Here's how the part is built. I have some questions about the finished solid (model axes, mm). Face numbers are marked on the shaded views. A direction names the side the tool comes from. Round coordinates to 2 decimals unless told otherwise and drop trailing zeros. Order: outer loops, then holes, each group sorted by start corner. A loop starts at its lowest first (then second) coordinate and runs counter-clockwise, first axis right, second up. Notation, with made-up numbers: M 22,-32.75 L 72,-32.75 A25 cw 72,-9.75 Z; hole C -7.5,46.5 d4. An arc over 180 degrees is marked long. Write item = value, one per line. Start each with the question number.
Item 1: I want a section at C-C, the plane x = -14.5. List the corners of the cut face in (y, z) for me, plus the area to 3 significant figures.
Item 2: I want a section at A-A, the plane x = 29. List the corners of the cut face in (y, z) for me, plus the area to 3 significant figures.
Item 3: I'm going to push flat-ended pins straight in: P1, Ø5, axis at x = -9.5, z = -7, coming from the +Y side; P2, Ø5, axis at y = -4, z = -5, coming from the +X side; P3, Ø0.5, axis at x = 25.5, y = 0, coming from the -Z side; P4, Ø8, axis at y = -29, z = -3, coming from the -X side. Where does each tip first touch, or does it pass through?
Item 4: We'd pull the mould along Y, two halves only. Please class the marked faces 4, 5 and 6: pulls with the +Y half, pulls with the -Y half, needs draft (parallel to the pull), parting line crosses it, or undercut.
Item 5: I want a section at D-D, the plane y = -20. List the corners of the cut face in (x, z) for me.
Item 6: For the marked faces 1, 2 and 3, which set-ups out of +Z, -Z, +X, -X, +Y, -Y let a thin tool reach every point of the face, with its end or its side?
Item 7: Please list where these lines run through material, in increasing order: L1, parallel to Y at x = -24, z = -5.5; L2, parallel to X at y = 0, z = -7.5; L3, parallel to Z at x = 26, y = 0.
Item 8: I want a section at B-B, the plane z = -2.75. List the corners of the cut face in (x, y) for me.
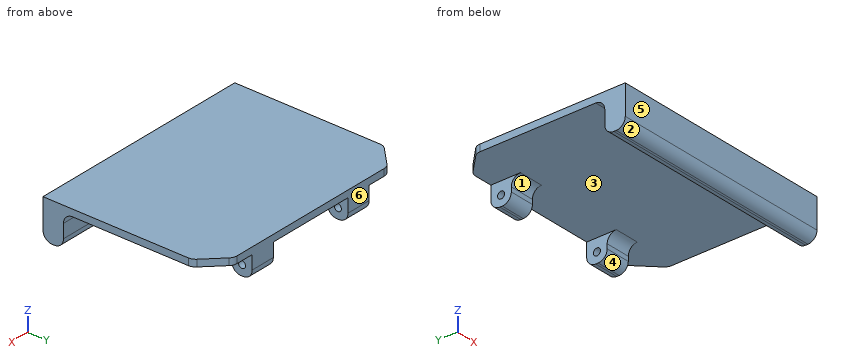
Autodesk Inventor part; units mm, degrees
ref_plane "YZ Plane" through (0, 0, 0) normal (1, 0, 0) x (0, 1, 0)
ref_plane "XZ Plane" through (0, 0, 0) normal (0, 1, 0) x (-1, 0, 0)
ref_plane "XY Plane" through (0, 0, 0) normal (0, 0, 1) x (1, 0, 0)
sketch "Sketch1" plane through (0, 0, 0) normal (0, 0, 1) x (1, 0, 0)
  line L0 (-30.5, 4.5) -> (-19.5, 4.5)
  line L1 (-19.5, 4.5) -> (-19.5, -4.5)
  line L2 (-19.5, -4.5) -> (-30.5, -4.5)
  line L3 (-30.5, -4.5) -> (-30.5, 4.5)
  line L4 (19.5, 4.5) -> (30.5, 4.5)
  line L5 (30.5, 4.5) -> (30.5, -4.5)
  line L6 (30.5, -4.5) -> (19.5, -4.5)
  line L7 (19.5, -4.5) -> (19.5, 4.5)
  line L8 (-50, 4.5) -> (50, 4.5)
  line L9 (50, 4.5) -> (50, -71)
  line L10 (50, -71) -> (-50, -71)
  line L11 (-50, -71) -> (-50, 4.5)
  point P0 (0, 0)
  dimension "d0" = 11
  dimension "d1" = 9
  dimension "d2" = 19.5
  dimension "d3" = 4.5
  dimension "d4" = 11
  dimension "d5" = 19.5
  dimension "d6" = 9
  dimension "d7" = 100
  dimension "d8" = 50
  dimension "d9" = 4.5
  dimension "d10" = 71
extrude "Extrusion1" add sketch "Sketch1" along normal blind 3
extrude "Extrusion2" add sketch "Sketch1" against normal blind 10 contours L0 L1 L2 L3 | L4 L5 L6 L7
sketch "Sketch2" plane through (30.5, -4.5, 0) normal (1, 0, 0) x (0, 0, -1)
  line L0 (0, 0) -> (0, 9)
  line L1 (0, 0) -> (10, 0)
  line L2 (10, 9) -> (10, 0)
  line L3 (0, 9) -> (10, 9)
  point P0 (0, 4.5)
  point P1 (5.5, 4.5)
  dimension "d15" = 4.5
  dimension "d16" = 4.5
hole "Hole1" at (30.5, 0, -5.5) direction (-1, 0, 0) diameter 3.1 end through all
fillet "Fillet1" radius 4 6 edges at (25, 4.5, -10) (25, -4.5, -10) (-25, -4.5, -10) (-25, 4.5, -10) (-25, -4.5, 0) (25, -4.5, 0)
chamfer "Chamfer1" distance 10 angle 45 2 edges at (50, 4.5, 1.5) (-50, 4.5, 1.5)
sketch "Sketch3" plane through (0, 0, 0) normal (0, 0, -1) x (-1, 0, 0)
  line L0 (40, 4.5) -> (50, -5.5)
  line L1 (30.5, 4.5) -> (40, 4.5)
  line L2 (30.5, 4.5) -> (30.5, -8.5)
  line L3 (19.5, -8.5) -> (30.5, -8.5)
  line L4 (19.5, -8.5) -> (19.5, 4.5)
  line L5 (-19.5, 4.5) -> (19.5, 4.5)
  line L6 (-19.5, 4.5) -> (-19.5, -8.5)
  line L7 (-30.5, -8.5) -> (-19.5, -8.5)
  line L8 (-30.5, -8.5) -> (-30.5, 4.5)
  line L9 (-40, 4.5) -> (-30.5, 4.5)
  line L10 (-50, -5.5) -> (-40, 4.5)
  line L11 (-50, -71) -> (-50, -5.5)
  line L12 (50, -71) -> (-50, -71)
  line L13 (50, -5.5) -> (50, -71)
  line L14 (-50, -62) -> (50, -62)
  point P0 (0, 0)
  dimension "d28" = 9
extrude "Extrusion3" add sketch "Sketch3" along normal blind 14 contours L13 L12 L11 L14
fillet "Fillet2" radius 4 3 edges at (0, -71, -14) (0, -62, -14) (0, -62, 0)
fillet "Fillet3" radius 4 4 edges at (-50, -5.5, 1.5) (-40, 4.5, 1.5) (40, 4.5, 1.5) (50, -5.5, 1.5)
equation "\"d4\" = d0"
properties part number "3DP_PLA_Stand_Leg"
Filled in:
q1.outline = M -71,-10 A4 ccw -67,-14 L -66,-14 A4 ccw -62,-10 L -62,-4 A4 cw -58,0 L 4.5,0 L 4.5,3 L -71,3 Z
q1.area = 349 mm^2
q2.outline = M -71,-10 A4 ccw -67,-14 L -66,-14 A4 ccw -62,-10 L -62,-4 A4 cw -58,0 L -8.5,0 A4 cw -4.5,-4 L -4.5,-6 A4 ccw -0.5,-10 L 0.5,-10 A4 ccw 4.5,-6 L 4.5,3 L -71,3 Z; hole C 0,-5.5 d3.1
q2.area = 428 mm^2
q3.P1 = -62
q3.P2 = 30.5
q3.P3 = -10
q3.P4 = -50
q4.face_4 = undercut
q4.face_5 = pulls with the -Y half
q4.face_6 = pulls with the +Y half
q5.outline = M -50,0 L 50,0 L 50,3 L -50,3 Z
q6.face_1 = -Z, +X, -X
q6.face_2 = -Z, +X, -X, -Y
q6.face_3 = -Z
q7.L1 = -71 to -62, -4.5 to -1.55, 1.55 to 4.5
q7.L2 = -30.5 to -19.5, 19.5 to 30.5
q7.L3 = -10 to -7.05, -3.95 to 3
q8.outline = M -50,-71 L 50,-71 L 50,-61.8 L -50,-61.8 Z; M -30.5,-4.7 L -19.5,-4.7 L -19.5,4.5 L -30.5,4.5 Z; M 19.5,-4.7 L 30.5,-4.7 L 30.5,4.5 L 19.5,4.5 Z
